from build123d import *

# Parameters (mm, degrees)
SKETCH4_R           = 1.225
SKETCH4_R_2         = 0.56
BOSS_EXTRUDE1_DEPTH = 32
BOSS_EXTRUDE2_DEPTH = 1.225
SKETCH5_R           = 0.56
CUT_EXTRUDE1_DEPTH  = 32
FILLET1_R           = 1


with BuildPart() as part:
    # Sketch4 → Boss-Extrude1 (new body)
    with BuildSketch(Plane(origin=(24.384171153, 175.5596446, 0), x_dir=(-0.990491591, 0.137573282, 0), z_dir=(-0.137573282, -0.990491591, 0))):
        with Locations((15.494896665, 0)):
            Circle(SKETCH4_R)
        with Locations((15.494896665, 0)):
            Circle(SKETCH4_R_2, mode=Mode.SUBTRACT)
    extrude(amount=-BOSS_EXTRUDE1_DEPTH)

    # Sketch2 → Boss-Extrude2 (add, symmetric)
    with BuildSketch(Plane.XY):
        Polygon((-9.272942535, 193.66488497), (11.829402487, 209.610615887), (7.427057465, 177.91488497), (-9.272942535, 177.91488497), align=None)
        Polygon((9.036606301, 177.691328387), (13.438951323, 209.387059303), (11.829402487, 209.610615887), (7.427057465, 177.91488497), align=None)
    extrude(amount=BOSS_EXTRUDE2_DEPTH, both=True)

    # Sketch5 → Cut-Extrude1 (cut)
    with BuildSketch(Plane(origin=(24.384171153, 175.5596446, 0), x_dir=(0.990491591, -0.137573282, 0), z_dir=(-0.137573282, -0.990491591, 0))):
        with Locations((-15.494896665, 0)):
            Circle(SKETCH5_R)
    extrude(amount=-CUT_EXTRUDE1_DEPTH, mode=Mode.SUBTRACT)

    # Fillet1
    fillet1_edges = [part.edges().sort_by_distance(p)[0] for p in [
        (1.278229976, 201.637750428, 1.225),
        (11.829402487, 209.610615887, 0),
        (-9.272942535, 185.78988497, 1.225),
        (-9.272942535, 193.66488497, 0),
        (-9.272942535, 177.91488497, 0),
        (1.278229976, 201.637750428, -1.225),
        (-9.272942535, 185.78988497, -1.225),
    ]]
    fillet(fillet1_edges, radius=FILLET1_R)


solid = part.part
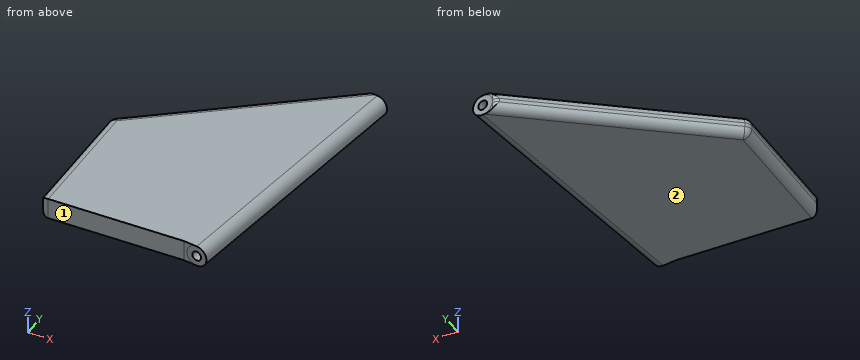
Work out the finished part from the listing and answer in its coordinate system (mm). Face numbers are marked on the shaded views. A direction names the side the tool comes from. Give positions to 0.01 mm unless a question says otherwise; leave off trailing zeros. Answer in a Markdown table with one row per item. Add a question column.
Q1. A tool of negligible diameter and unlimited length cuts with its end or side. For the marked faces 1 and 2, from which of +Z, -Z, +X, -X, +Y, -Y can it reach the whole face along a straight path? Write none if from no direction.
Q2. This flat-tipped pin is pushed along its axis until it touches: P1, Ø1, axis at x = 5, z = -0.5, coming from the -Y side. Where does it stop, or does it pass through?
Q3. Consider line 1 along X through (y, z) = (198.5, -0.45); line 2 along Z through (x, y) = (10.75, 189); line 3 along X through (y, z) = (190, 0.1). Determine where each line is inside the solid, lowest interval first.
Solution:
| question | item | result |
|---|---|---|
| 1 | face 1 | +Z, -Z, -X, -Y |
| 1 | face 2 | -Z, +X, -X, +Y, -Y |
| 2 | P1 | stops at y = 177.91 |
| 3 | line 1 | x = -2.83 to 11.59, 12.26 to 13.08 |
| 3 | line 2 | z = -1.22 to -0.54, 0.54 to 1.22 |
| 3 | line 3 | x = -9.27 to 10.19, 11.3 to 11.98 |
